from build123d import *

# Parameters (mm, degrees)
BOSS_EXTRU_1_DEPTH      = 5
ESQUISSE2_R             = 17
ENL_V_MAT_EXTRU_1_DEPTH = 162.632298752


with BuildPart() as part:
    # Esquisse1 → Boss.-Extru.1 (new body)
    with BuildSketch(Plane.XY):
        Polygon((-90, 60), (-150, 60), (-150, 15), (-145, 15), (-145, 1.5), (-141.5, 1.5), (-141.5, 2.5), (-138.5, 2.5), (-138.5, 1.5), (-135, 1.5), (-135, -1.5), (-138.5, -1.5), (-138.5, -2.5), (-141.5, -2.5), (-141.5, -1.5), (-145, -1.5), (-145, -15), (-150, -15), (-150, -60), (-90, -60), (-60, -60), (60, -60), (90, -60), (150, -60), (150, -15), (145, -15), (145, -1.5), (141.5, -1.5), (141.5, -2.5), (138.5, -2.5), (138.5, -1.5), (135, -1.5), (135, 1.5), (138.5, 1.5), (138.5, 2.5), (141.5, 2.5), (141.5, 1.5), (145, 1.5), (145, 15), (150, 15), (150, 60), (90, 60), (90, 55), (76.5, 55), (76.5, 51.5), (77.5, 51.5), (77.5, 48.5), (76.5, 48.5), (76.5, 45), (73.5, 45), (73.5, 48.5), (72.5, 48.5), (72.5, 51.5), (73.5, 51.5), (73.5, 55), (60, 55), (60, 60), (-60, 60), (-60, 55), (-73.5, 55), (-73.5, 51.5), (-72.5, 51.5), (-72.5, 48.5), (-73.5, 48.5), (-73.5, 45), (-76.5, 45), (-76.5, 48.5), (-77.5, 48.5), (-77.5, 51.5), (-76.5, 51.5), (-76.5, 55), (-90, 55), align=None)
    extrude(amount=BOSS_EXTRU_1_DEPTH)

    # Esquisse2 → Enlèv. mat.-Extru.1 (cut, through all)
    with BuildSketch(Plane(origin=(0, 0, 0), x_dir=(-1, 0, 0), z_dir=(0, 0, -1))):
        with Locations((0, 5)):
            Circle(ESQUISSE2_R)
    extrude(amount=-ENL_V_MAT_EXTRU_1_DEPTH, mode=Mode.SUBTRACT)


solid = part.part
CAD build for the part. Positions are in the model's coordinates, mm. A direction names the side the tool comes from. Round coordinates to 2 decimals unless told otherwise and drop trailing zeros. Order: outer loops, then holes, each group sorted by start corner. A loop starts at its lowest first (then second) coordinate and runs counter-clockwise, first axis right, second up. Notation, with made-up numbers: (18.25, -3) -> (51.25, -3) arc R27 ccw to (51.25, 14) -> close; hole circle Ø7 at (73.5, 26). An arc over 180 degrees is marked (long way). Write item = value, one per line. Start each with the question number.
(1) Pull direction Y, two halves, no side cores. Call faces 5 (the flat face through (60, 57, 2)), 6 (the flat face through (-2, -60, 2)), 7 (the flat face through (-147, -15, 2)), 8 (the flat face through (67, 55, 2)): released by +Y, released by -Y, zero draft, split by the parting line, or undercut.
(2) Probe line 1 (X direction, y = 49.5, z = 3.6); line 2 (Y direction, x = 0, z = 2.4); line 3 (Y direction, x = 65, z = 1.85). List the from-to ranges inside material, lowest first. Write a range as [from, to].
(3) Cut at C-C, the plane x = -83.5. List the corners of the cut face in (y, z).
(4) Which spindle directions (+Z, -Z, +X, -X, +Y, -Y) get a long thin tool onto all of the face, cutting with end or side? Do faces 1 (the flat face through (145, -8, 2)), 2 (the flat face through (150, 37, 2)), 3 (the flat face through (-67, 55, 2)), 4 (the flat face through (-145, -8, 2)). Say none if no direction does.
(5) Cut at B-B, the plane y = 10. List the corners of the cut face in (x, z).
(6) Pin check, flat tips, straight feed: P1, Ø0.5, axis at y = -2, z = 2, coming from the +X side; P2, Ø2, axis at y = -9, z = 2, coming from the -X side; P3, Ø2.5, axis at x = 85.5, z = 2, coming from the +Y side. Stop position of each tip, or through.
(7) Cut at A-A, the plane x = 0. List the corners of the cut face in (y, z).
Model answer:
q1.face_5 = zero draft
q1.face_6 = released by -Y
q1.face_7 = undercut
q1.face_8 = released by +Y
q2.line_1 = [-150, -77.5], [-72.5, 72.5], [77.5, 150]
q2.line_2 = [-60, -12], [22, 60]
q2.line_3 = [-60, 55]
q3.outline = (-60, 0) -> (55, 0) -> (55, 5) -> (-60, 5) -> close
q4.face_1 = +Z, -Z, +X
q4.face_2 = +Z, -Z, +X, +Y, -Y
q4.face_3 = +Z, -Z, +Y
q4.face_4 = +Z, -Z, -X
q5.outline = (-145, 0) -> (-16.25, 0) -> (-16.25, 5) -> (-145, 5) -> close; (16.25, 0) -> (145, 0) -> (145, 5) -> (16.25, 5) -> close
q6.P1 = 145
q6.P2 = -145
q6.P3 = 55
q7.outline = (-60, 0) -> (-12, 0) -> (-12, 5) -> (-60, 5) -> close; (22, 0) -> (60, 0) -> (60, 5) -> (22, 5) -> close
